Job drawing, mm, ordinate dimensions from the low corner. One solid piece. A direction names the side the tool comes from. Give positions to 0.01 mm unless a question says otherwise; leave off trailing zeros. Order: outer loops, then holes, each group sorted by start corner. A loop starts at its lowest first (then second) coordinate and runs counter-clockwise, first axis right, second up.
Item 1: Wall check: L1, parallel to Y at x = 39, z = 90.5; L2, parallel to Z at x = 65, y = 54; L3, parallel to X at y = 30.25, z = 87 (1 decimal). Give the ranges that are in metal, low to high.
Item 2: Band-saw the part on C-C on z = 42.5. Give the cut face in (x, y), plus the area to 3 significant figures.
Item 3: Flat gauge pins, fed straight in: P1, Ø12, axis at x = 29.5, z = 13, coming from the -Y side; P2, Ø4, axis at x = 54.16, y = 30.25, coming from the -Z side; P3, Ø1, axis at x = 63.5, z = 76, coming from the +Y side; P4, Ø3, axis at x = 11, z = 22.5, coming from the -Y side (1 decimal). Where does each tip first touch, or does it go through?
Item 4: Which spindle directions (+Z, -Z, +X, -X, +Y, -Y) get a long thin tool onto all of the face, cutting with end or side? Do the marked faces 1 and 2. Say none if no direction does.
Item 5: Band-saw the part on B-B on x = 16. Give the cut face in (y, z).
Item 6: Band-saw the part on D-D on y = 72.5. Give the cut face in (x, z).
Item 7: Band-saw the part on A-A on y = 39. Give the cut face in (x, z), plus the area to 3 significant figures.
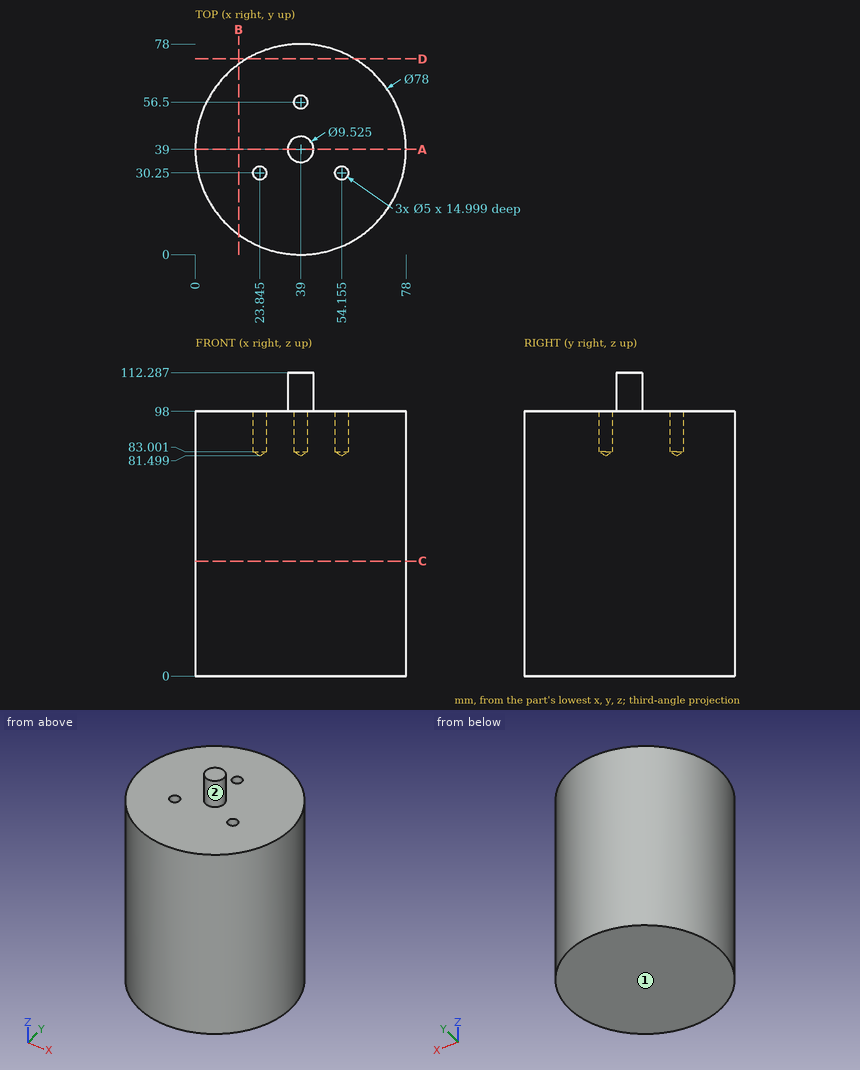
The answers:
1. L1: y = 0 to 54, 59 to 78
1. L2: z = 0 to 98
1. L3: x = 1 to 21.3, 26.3 to 51.7, 56.7 to 77
2. outline: circle Ø78 at (39, 39)
2. area: 4,780 mm2
3. P1: stops at y = 0.16
3. P2: stops at z = 0
3. P3: stops at y = 69.74
3. P4: stops at y = 10.4
4. face 1: -Z, +X, -X, +Y, -Y
4. face 2: +Z
5. outline: (7.5, 0) - (70.5, 0) - (70.5, 98) - (7.5, 98) - close
6. outline: (19.03, 0) - (58.97, 0) - (58.97, 98) - (19.03, 98) - close
7. outline: (0, 0) - (78, 0) - (78, 98) - (43.76, 98) - (43.76, 112.29) - (34.24, 112.29) - (34.24, 98) - (0, 98) - close
7. area: 7,780 mm2
